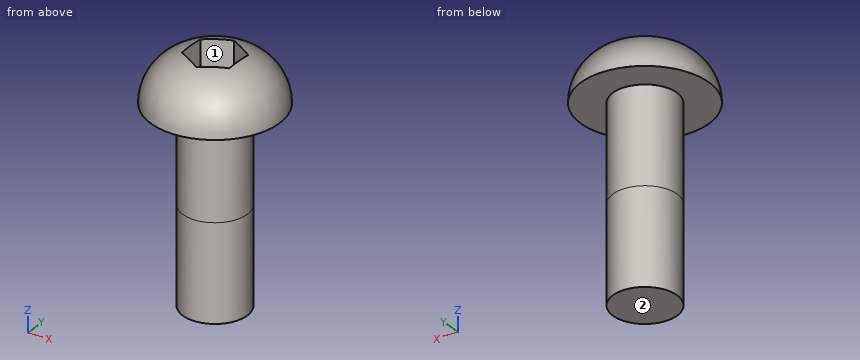
Autodesk Inventor part; units mm, degrees
ref_plane "YZ Plane" through (0, 0, 0) normal (1, 0, 0) x (0, 1, 0)
ref_plane "XZ Plane" through (0, 0, 0) normal (0, 1, 0) x (-1, 0, 0)
ref_plane "XY Plane" through (0, 0, 0) normal (0, 0, 1) x (1, 0, 0)
sketch "スケッチ1" plane through (0, 0, 0) normal (0, 0, 1) x (1, 0, 0)
  circle A0 centre (0, 0) radius 2
  dimension "d0" = 4
extrude "押し出し1" add sketch "スケッチ1" along normal blind 6
sketch "スケッチ2" plane through (0, 0, 6) normal (0, 0, 1) x (1, 0, 0)
  circle A0 centre (0, 0) radius 2
  circle A1 centre (0, 0) radius 4
  dimension "d3" = 8
extrude "押し出し2" add sketch "スケッチ2" along normal blind 3 contours A0 | A1
fillet "フィレット1" radius 3 1 edges at (-4, 0, 9)
thread "ねじ1"
sketch "スケッチ3" plane through (0, 0, 0) normal (0, 0, -1) x (-1, 0, 0)
  circle A0 centre (0, 0) radius 2
extrude "押し出し3" add sketch "スケッチ3" along normal blind 6
sketch "スケッチ4" plane through (0, 0, 9) normal (0, 0, 1) x (1, 0, 0)
  line L0 (-1.5, 0.866) -> (0, 1.7321)
  line L1 (0, 1.7321) -> (1.5, 0.866)
  line L2 (1.5, 0.866) -> (1.5, -0.866)
  line L3 (1.5, -0.866) -> (0, -1.7321)
  line L4 (0, -1.7321) -> (-1.5, -0.866)
  line L5 (-1.5, -0.866) -> (-1.5, 0.866)
  point P0 (0, 0)
  point P1 (0, 0)
  point P2 (-1.5, 0)
  dimension "d11" = 3
extrude "押し出し4" cut sketch "スケッチ4" against normal blind 2
properties part number "SB　M4 12mm なべネジ (1)" material "Stainless Steel, 440C"
Work out the finished part from the listing and answer in its coordinate system (mm). Face numbers are marked on the shaded views. Coordinates: 2 decimals unless noted, no trailing zeros. Write each loop counter-clockwise with the first axis right and the second up, starting at its lowest first coordinate (ties: lowest second). Pieces come first, ordered by that corner, then holes. Notation, with made-up numbers: M -0.75,30 L 42.25,30 A4 ccw 42.25,36 Z; hole C 77.25,75 d5. An arc over 180 degrees is marked long. Answer as CSV lines item,"result". Start each with the question number.
Item 1: Flat-ended cylindrical pins translate along their axes: P1, Ø1.4, axis at y = 0, z = 8, coming from the -X side; P2, Ø2, axis at y = 0, z = 2, coming from the +X side; P3, Ø1.5, axis at x = -0.5, y = 0, coming from the +Z side. Find the tip coordinate at first contact, or state that the pin passes through.
Item 2: Consider L1, parallel to Z at x = -1, y = 0.75; L2, parallel to X at y = 0, z = 3.75; L3, parallel to Y at x = 0.25, z = 7.5. Determine where each line is inside the solid, lowest interval first.
Item 3: Determine the mould class of the marked faces 1 and 2 for opening direction X: released by +X, released by -X, zero draft, split by the parting line, or undercut.
Item 4: Section A-A on z = -1.75 is taken. Write down the section's boundary in (x, y), and give its area (3 significant figures).
Checks:
1,P1,"stops at x = -3.7"
1,P2,"stops at x = 2"
1,P3,"stops at z = 7"
2,L1,"z = -6 to 7"
2,L2,"x = -2 to 2"
2,L3,"y = -3.59 to -1.59, 1.59 to 3.59"
3,face 1,"undercut"
3,face 2,"zero draft"
4,outline,"C 0,0 d4"
4,area,"12.6 mm²"
